Check sheet for the modelled part. Datum: model origin and axes. Units: mm. Round coordinates to 2 decimals unless told otherwise and drop trailing zeros. Write each loop counter-clockwise with the first axis right and the second up, starting at its lowest first coordinate (ties: lowest second). Pieces come first, ordered by that corner, then holes. Notation, with made-up numbers: (-7, 27) - (36, 27) arc R23 ccw to (36, 37) - close; hole circle Ø7 at (19, 20.25). An arc over 180 degrees is marked (long way). Answer as a JSON object with one key per item and string values. Group by question number.
Item 1: Gauge pin test, flat ends, axial feed: P1, Ø6, axis at x = 1049.5, y = -10, coming from the -Z side; P2, Ø1.5, axis at y = 38.5, z = 1, coming from the -X side; P3, Ø1.5, axis at x = 1050.5, z = 1, coming from the -Y side; P4, Ø0.9, axis at x = 1014.5, z = 2, coming from the +Y side. Record the tip position at first contact, or that the pin passes through.
Item 2: Sectioned sample at A-A on y = -47. Record the boundary of the cut face in (x, z).
Item 3: Thickness scan on line 1 (X direction, y = -48.5, z = 0.25); line 2 (X direction, y = 16.5, z = 1.35); line 3 (X direction, y = -50, z = 2.05). Record the ranges inside material, lowest first.
Item 4: Sectioned sample at B-B on x = 1036.5. Record the boundary of the cut face in (y, z).
Item 5: Sectioned sample at C-C on z = 2.15. Count the separate pieces of the cut face and the enclosed holes in it, plus the area to 3 significant figures.
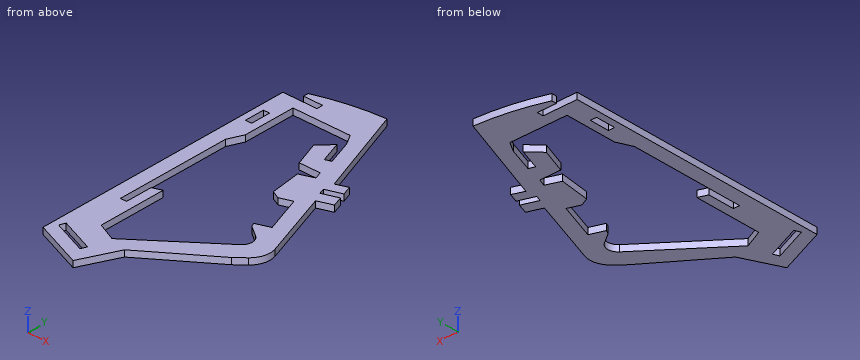
```python
from build123d import *

# Parameters (mm, degrees)
SKETCH1_W           = 3
SKETCH1_H           = 9.45
BASE_EXTRUDE_DEPTH  = 3
SKETCH2_W           = 10
SKETCH2_H           = 3
BOSS_EXTRUDE1_DEPTH = 3


with BuildPart() as part:
    # Sketch1 → Base-Extrude (new body)
    with BuildSketch(Plane.XY):
        with BuildLine():
            Line((1079.876919763, -44.105153511), (1068.056216666, -10.172974917))
            Line((1068.056216666, -10.172974917), (1074.996757052, -7.75514999))
            Line((1074.996757052, -7.75514999), (1073.279825248, -2.753207543))
            Line((1073.279825248, -2.753207543), (1065.713177122, -5.350482293))
            Line((1065.713177122, -5.350482293), (1064.73919909, -2.512989245))
            Line((1064.73919909, -2.512989245), (1072.305847217, 0.084285505))
            Line((1072.305847217, 0.084285505), (1070.719575987, 4.705574119))
            Line((1070.719575987, 4.705574119), (1065.157526034, 2.696840543))
            Line((1065.157526034, 2.696840543), (1048.759611565, 48.101577381))
            ThreePointArc((1048.759611565, 48.101577381), (1032.39485012, 46.101647559), (1016.466345621, 41.848662618))
            Line((1016.466345621, 41.848662618), (1016.466345621, 39.392602571))
            Line((1016.466345621, 39.392602571), (1035.726137056, 39.392602571))
            Line((1035.726137056, 39.392602571), (1035.726137056, 36.392602571))
            Line((1035.726137056, 36.392602571), (1009.279499751, 36.392602571))
            Line((1009.279499751, 36.392602571), (1009.279499751, -89.073987735))
            Line((1009.279499751, -89.073987735), (1032.543515661, -98.536722682))
            Line((1032.543515661, -98.536722682), (1040.991113984, -80.770341528))
            Line((1040.991113984, -80.770341528), (1072.440441541, -58.876157059))
            Line((1072.440441541, -58.876157059), (1076.9710582, -54.961956755))
            ThreePointArc((1076.9710582, -54.961956755), (1080.093496996, -49.980404823), (1079.876919763, -44.105153511))
        make_face()
        with BuildLine():
            Line((1019.213878108, 30.925856164), (1019.213878108, 6.018771541))
            Line((1019.213878108, 6.018771541), (1016.100082492, -1.038872257))
            Line((1016.100082492, -1.038872257), (1016.100082492, -55.976738358))
            Line((1016.100082492, -55.976738358), (1019.100082492, -55.976738358))
            Line((1019.100082492, -55.976738358), (1019.100082492, -43.198135443))
            Line((1019.100082492, -43.198135443), (1023.478597046, -41.580404808))
            Line((1023.478597046, -41.580404808), (1023.478597046, -73.992128786))
            Line((1023.478597046, -73.992128786), (1032.526582577, -78.167039678))
            Line((1032.526582577, -78.167039678), (1068.850484509, -50.258348586))
            ThreePointArc((1068.850484509, -50.258348586), (1070.803657728, -46.221334872), (1068.734776871, -42.242378056))
            Line((1068.734776871, -42.242378056), (1063.325122863, -38.329012558))
            Line((1063.325122863, -38.329012558), (1062.407393196, -36.386031272))
            Line((1062.407393196, -36.386031272), (1069.115709638, -34.04910449))
            Line((1069.115709638, -34.04910449), (1062.700744223, -15.634484789))
            Line((1062.700744223, -15.634484789), (1056.810312455, -17.686491112))
            Line((1056.810312455, -17.686491112), (1052.869598475, -15.779326268))
            Line((1052.869598475, -15.779326268), (1050.941521122, -1.083078235))
            Line((1050.941521122, -1.083078235), (1057.625060998, 1.362146575))
            Line((1057.625060998, 1.362146575), (1056.321001716, 4.948397029))
            Line((1056.321001716, 4.948397029), (1046.214175082, 4.948397029))
            Line((1046.214175082, 4.948397029), (1041.773169547, 17.294470752))
            Line((1041.773169547, 17.294470752), (1047.600835278, 23.111994965))
            Line((1047.600835278, 23.111994965), (1051.253809923, 12.605592538))
            Line((1051.253809923, 12.605592538), (1054.100349004, 13.552807012))
            Line((1054.100349004, 13.552807012), (1049.909104568, 25.720739733))
            Line((1049.909104568, 25.720739733), (1046.816291402, 30.939914406))
            Line((1046.816291402, 30.939914406), (1019.213878108, 30.925856164))
        make_face(mode=Mode.SUBTRACT)
        Polygon((1012.307844389, -84.207250741), (1013.438177941, -81.428339792), (1030.025357256, -88.175243766), (1028.895023704, -90.954154714), align=None, mode=Mode.SUBTRACT)
        with Locations((1013.982987836, 18.006853638)):
            Rectangle(SKETCH1_W, SKETCH1_H, mode=Mode.SUBTRACT)
    extrude(amount=BASE_EXTRUDE_DEPTH)

    # Sketch2 → Boss-Extrude1 (add)
    with BuildSketch(Plane.XY.offset(3)):
        with Locations((1030.726137056, 37.892602571)):
            Rectangle(SKETCH2_W, SKETCH2_H)
    extrude(amount=-BOSS_EXTRUDE1_DEPTH)


solid = part.part
```
Completed:
{
 "1": {"P1": "z = 0", "P2": "x = 1025.73", "P3": "y = -74.67", "P4": "y = 36.39"},
 "2": {"outline": "(1009.28, 0) - (1016.1, 0) - (1016.1, 3) - (1009.28, 3) - close; (1019.1, 0) - (1023.48, 0) - (1023.48, 3) - (1019.1, 3) - close; (1070.75, 0) - (1080.43, 0) - (1080.43, 3) - (1070.75, 3) - close"},
 "3": {"line 1": "1009.28 to 1016.1, 1019.1 to 1023.48, 1070.29 to 1080.37", "line 2": "1009.28 to 1012.48, 1015.48 to 1019.21, 1042.06 to 1049.9, 1053.09 to 1060.17", "line 3": "1009.28 to 1016.1, 1019.1 to 1023.48, 1069.16 to 1080.09"},
 "4": {"outline": "(-90.22, 0) - (-75.11, 0) - (-75.11, 3) - (-90.22, 3) - close; (30.93, 0) - (46.82, 0) - (46.82, 3) - (30.93, 3) - close"},
 "5": {"separate pieces": "1", "enclosed holes": "3", "area": "3,390 mm²"}
}
